Model file for the job. Use its own axes, mm. Face numbers are marked on the shaded views. A direction names the side the tool comes from. Coordinates: 2 decimals unless noted, no trailing zeros. Loops run counter-clockwise (first coordinate to the right, second up) from the corner with the lowest first, then second, coordinate; pieces in that order, holes last.
from build123d import *

# Parameters (mm, degrees)
SKETCH_1_R          = 32.5
SKETCH_1_R_2        = 21.5
EXTRUDE_1_DEPTH     = 4
SKETCH_2_R          = 30
SKETCH_2_R_2        = 21.5
EXTRUDE_2_DEPTH     = 15
SKETCH_3_R          = 2
CUT_EXTRUDE_1_DEPTH = 50.734294003


with BuildPart() as part:
    # 草图1 → 凸台-拉伸1 (new body)
    with BuildSketch(Plane.XY):
        Circle(SKETCH_1_R)
        Circle(SKETCH_1_R_2, mode=Mode.SUBTRACT)
    extrude(amount=EXTRUDE_1_DEPTH)

    # 草图2 → 凸台-拉伸2 (add)
    with BuildSketch(Plane.XY.offset(4)):
        Circle(SKETCH_2_R)
        Circle(SKETCH_2_R_2, mode=Mode.SUBTRACT)
    extrude(amount=EXTRUDE_2_DEPTH)

    # 草图3 → 切除-拉伸1 (cut, through all)
    with BuildSketch(Plane(origin=(0, 0, 0), x_dir=(-1, 0, 0), z_dir=(0, 0, -1))):
        with Locations((18.03122292, 18.03122292)):
            Circle(SKETCH_3_R)
        with Locations((25.5, 0)):
            Circle(SKETCH_3_R)
        with Locations((18.03122292, -18.03122292)):
            Circle(SKETCH_3_R)
        with Locations((0, -25.5)):
            Circle(SKETCH_3_R)
        with Locations((-18.03122292, -18.03122292)):
            Circle(SKETCH_3_R)
        with Locations((-25.5, 0)):
            Circle(SKETCH_3_R)
        with Locations((-18.03122292, 18.03122292)):
            Circle(SKETCH_3_R)
        with Locations((0, 25.5)):
            Circle(SKETCH_3_R)
        with BuildLine():
            ThreePointArc((7.613529763, 26.945021146), (10.715136106, 25.86862691), (13.669428647, 24.436585696))
            ThreePointArc((13.669428647, 24.436585696), (14.630781955, 21.034262987), (11.228459246, 20.072909679))
            ThreePointArc((11.228459246, 20.072909679), (8.801718944, 21.249229248), (6.253970877, 22.133410227))
            ThreePointArc((6.253970877, 22.133410227), (4.527944861, 25.218995129), (7.613529763, 26.945021146))
        make_face()
        with BuildLine():
            ThreePointArc((24.436585696, 13.669428647), (21.034262987, 14.630781955), (20.072909679, 11.228459246))
            ThreePointArc((20.072909679, 11.228459246), (21.249229248, 8.801718944), (22.133410227, 6.253970877))
            ThreePointArc((22.133410227, 6.253970877), (25.218995129, 4.527944861), (26.945021146, 7.613529763))
            ThreePointArc((26.945021146, 7.613529763), (25.86862691, 10.715136106), (24.436585696, 13.669428647))
        make_face()
        with BuildLine():
            ThreePointArc((26.945021146, -7.613529763), (25.218995129, -4.527944861), (22.133410227, -6.253970877))
            ThreePointArc((22.133410227, -6.253970877), (21.249229248, -8.801718944), (20.072909679, -11.228459246))
            ThreePointArc((20.072909679, -11.228459246), (21.034262987, -14.630781955), (24.436585696, -13.669428647))
            ThreePointArc((24.436585696, -13.669428647), (25.86862691, -10.715136106), (26.945021146, -7.613529763))
        make_face()
        with BuildLine():
            ThreePointArc((13.669428647, -24.436585696), (14.630781955, -21.034262987), (11.228459246, -20.072909679))
            ThreePointArc((11.228459246, -20.072909679), (8.801718944, -21.249229248), (6.253970877, -22.133410227))
            ThreePointArc((6.253970877, -22.133410227), (4.527944861, -25.218995129), (7.613529763, -26.945021146))
            ThreePointArc((7.613529763, -26.945021146), (10.715136106, -25.86862691), (13.669428647, -24.436585696))
        make_face()
        with BuildLine():
            ThreePointArc((-7.613529763, -26.945021146), (-4.527944861, -25.218995129), (-6.253970877, -22.133410227))
            ThreePointArc((-6.253970877, -22.133410227), (-8.801718944, -21.249229248), (-11.228459246, -20.072909679))
            ThreePointArc((-11.228459246, -20.072909679), (-14.630781955, -21.034262987), (-13.669428647, -24.436585696))
            ThreePointArc((-13.669428647, -24.436585696), (-10.715136106, -25.86862691), (-7.613529763, -26.945021146))
        make_face()
        with BuildLine():
            ThreePointArc((-24.436585696, -13.669428647), (-21.034262987, -14.630781955), (-20.072909679, -11.228459246))
            ThreePointArc((-20.072909679, -11.228459246), (-21.249229248, -8.801718944), (-22.133410227, -6.253970877))
            ThreePointArc((-22.133410227, -6.253970877), (-25.218995129, -4.527944861), (-26.945021146, -7.613529763))
            ThreePointArc((-26.945021146, -7.613529763), (-25.86862691, -10.715136106), (-24.436585696, -13.669428647))
        make_face()
        with BuildLine():
            ThreePointArc((-26.945021146, 7.613529763), (-25.218995129, 4.527944861), (-22.133410227, 6.253970877))
            ThreePointArc((-22.133410227, 6.253970877), (-21.249229248, 8.801718944), (-20.072909679, 11.228459246))
            ThreePointArc((-20.072909679, 11.228459246), (-21.034262987, 14.630781955), (-24.436585696, 13.669428647))
            ThreePointArc((-24.436585696, 13.669428647), (-25.86862691, 10.715136106), (-26.945021146, 7.613529763))
        make_face()
        with BuildLine():
            ThreePointArc((-13.669428647, 24.436585696), (-14.630781955, 21.034262987), (-11.228459246, 20.072909679))
            ThreePointArc((-11.228459246, 20.072909679), (-8.801718944, 21.249229248), (-6.253970877, 22.133410227))
            ThreePointArc((-6.253970877, 22.133410227), (-4.527944861, 25.218995129), (-7.613529763, 26.945021146))
            ThreePointArc((-7.613529763, 26.945021146), (-10.715136106, 25.86862691), (-13.669428647, 24.436585696))
        make_face()
    extrude(amount=-CUT_EXTRUDE_1_DEPTH, mode=Mode.SUBTRACT)


solid = part.part
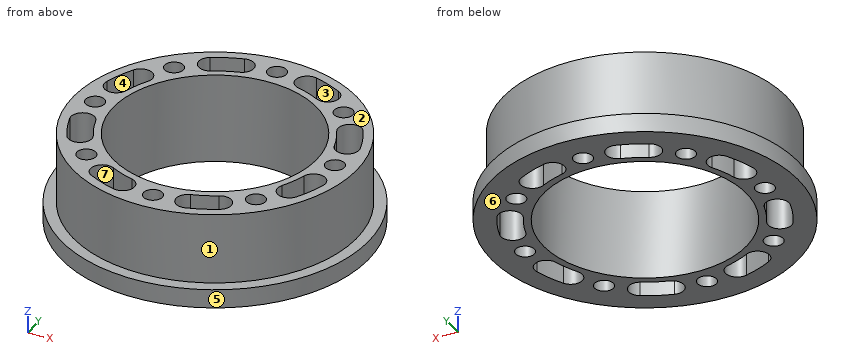
Q1. Slice it at C-C (z = 8.25). Count the separate pieces of the cut face and the enclosed holes in it, and give its area (3 significant figures).
Answers:
separate pieces: 1
enclosed holes: 17
area: 878 mm2
Q2. Drill centre lines: line 1 (Y direction, x = 0, z = 13.5); line 2 (X direction, y = 14.5, z = 18); line 3 (Y direction, x = -13, z = 10). Where is each one in solid material? Low to high.
Answers:
line 1: y = -30 to -27.5, -23.5 to -21.5, 21.5 to 23.5, 27.5 to 30
line 2: x = -26.26 to -23.68, -20.83 to -15.87, 15.87 to 20.83, 23.68 to 26.26
line 3: y = -27.04 to -24.8, -19.82 to -17.12, 17.12 to 19.82, 24.8 to 27.04
Q3. Slice it at A-A (y = 0). List the corners of the cut face in (x, z).
Answers:
outline: (-32.5, 0) - (-27.5, 0) - (-27.5, 19) - (-30, 19) - (-30, 4) - (-32.5, 4) - close; (-23.5, 0) - (-21.5, 0) - (-21.5, 19) - (-23.5, 19) - close; (21.5, 0) - (23.5, 0) - (23.5, 19) - (21.5, 19) - close; (27.5, 0) - (32.5, 0) - (32.5, 4) - (30, 4) - (30, 19) - (27.5, 19) - close
Q4. Which spindle directions (+Z, -Z, +X, -X, +Y, -Y) get a long thin tool onto all of the face, cutting with end or side? Do the marked faces 1, 2 and 3. Say none if no direction does.
Answers:
face 1: +Z
face 2: +Z, +X, -X, +Y, -Y
face 3: +Z, -Z
Q5. Mould opens along X. For the marked faces 4, 5, 6 and 7 say: +X half, -X half, draft (parallel to the pull), parting line (faces both ways), or undercut.
Answers:
face 4: undercut
face 5: parting line
face 6: draft
face 7: undercut
Q6. Flat gauge pins, fed straight in: P1, Ø2.5, axis at x = 25.5, y = 0, coming from the +Z side; P2, Ø8, axis at y = 5.5, z = 4.5, coming from the +X side; P3, Ø5, axis at y = 12.5, z = 16, coming from the -X side; P4, Ø4, axis at y = 11.5, z = 11, coming from the -X side. Where does each tip first touch, or does it go through?
Answers:
P1: passes through
P2: stops at x = 32.46
P3: stops at x = -28.28
P4: stops at x = -28.46
